Part model, mm, in its own coordinate system. Face numbers are marked on the shaded views. A direction names the side the tool comes from. Give positions to 0.01 mm unless a question says otherwise; leave off trailing zeros. Write each loop counter-clockwise with the first axis right and the second up, starting at its lowest first coordinate (ties: lowest second). Pieces come first, ordered by that corner, then holes. Notation, with made-up numbers: (-35.5, -25) - (21.5, -25) arc R25 ccw to (21.5, 11) - close; hole circle Ø3 at (-13.5, -28.5). An arc over 180 degrees is marked (long way). Answer as a JSON object with one key per item and string values. Group by question number.
```python
from build123d import *

# Parameters (mm, degrees)
SKETCH_1_R               = 20
EXTRUDE_1_DEPTH          = 5
SKETCH_1_7_R             = 3
EXTRUDE_2_DEPTH          = 10
SKETCH_2_R               = 0.75
CUT_EXTRUDE_1_DEPTH      = 31
PATTERN_CIRCULAR_1_COUNT = 6


with BuildPart() as part:
    # Sketch 1 → Extrude 1 (new body)
    with BuildSketch(Plane(origin=(0, 0, 0), x_dir=(1, 0, 0), z_dir=(0, 1, 0))):
        with Locations(Location((0, 0, 0), (0, 0, 270))):
            Circle(SKETCH_1_R)
    extrude(amount=EXTRUDE_1_DEPTH)

    # Sketch 1_7 → Extrude 2 (add)
    with BuildSketch(Plane(origin=(0, 0, 0), x_dir=(1, 0, 0), z_dir=(0, 1, 0))):
        with Locations(Location((0, 0, 0), (0, 0, 270))):
            Circle(SKETCH_1_7_R)
        with BuildLine():
            Line((-1, -1.118033989), (-1, 1.118033989))
            ThreePointArc((-1, 1.118033989), (1.5, 0), (-1, -1.118033989))
        make_face(mode=Mode.SUBTRACT)
    extrude(amount=EXTRUDE_2_DEPTH)

    # Sketch 2 → Cut-Extrude 1 (cut, through all)
    with BuildSketch(Plane.XZ):
        with Locations(Location((0, -7, 0), (0, 0, 270))):
            Circle(SKETCH_2_R)
        with Locations(Location((0, -17, 0), (0, 0, 270))):
            Circle(SKETCH_2_R)
    cut_extrude_1 = extrude(amount=-CUT_EXTRUDE_1_DEPTH, mode=Mode.SUBTRACT)

    # Pattern Circular 1: Cut-Extrude 1 ×6 about axis
    pattern_circular_1_axis = Axis((0, 0, 0), (0, 1, 0))
    for i in range(1, PATTERN_CIRCULAR_1_COUNT):
        add(cut_extrude_1.rotate(pattern_circular_1_axis, i * 360 / PATTERN_CIRCULAR_1_COUNT), mode=Mode.SUBTRACT)


solid = part.part
```
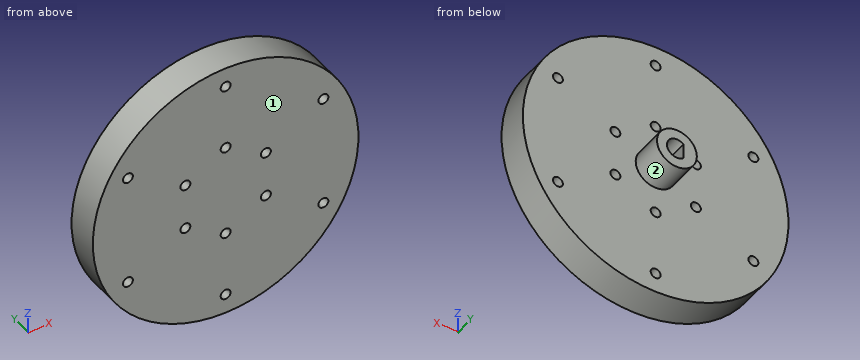
1) Saw through at D-D (z = -0.5). List the corners of the cut face in (x, y), and give its area (3 significant figures).
2) Drop flat-ended pins along their axis: P1, Ø5, axis at y = 5, z = -13.5, coming from the +X side; P2, Ø0.9, axis at x = 14.72, z = 8.5, coming from the -Y side; P3, Ø2, axis at x = -5, z = -8, coming from the +Y side; P4, Ø5, axis at x = -15, y = 5, coming from the +Z side. Give the stop position or say it passes through.
3) Saw through at B-B (y = 9.25). List the corners of the cut face in (x, z).
4) Drill centre lines: line 1 along Z through (x, y) = (0, 7.55); line 2 along X through (y, z) = (3.7, -8.5); line 3 along Y through (x, z) = (-8.5, 8.5). Where is each one in solid material? Low to high. Write a range as from..to.
5) Which spindle directions (+Z, -Z, +X, -X, +Y, -Y) get a long thin tool onto all of the face, cutting with end or side? Do the marked faces 1 and 2. Say none if no direction does.
6) Saw through at A-A (z = 7). List the corners of the cut face in (x, y) (3 decimals).
7) Saw through at C-C (y = 1.5). State how many separate pieces and enclosed holes the cut face has, and give its area (3 significant figures).
Checks:
{
 "1": {"outline": "(-19.99, 0) - (19.99, 0) - (19.99, 5) - (2.96, 5) - (2.96, 10) - (1.41, 10) - (1.41, 5) - (-1, 5) - (-1, 10) - (-2.96, 10) - (-2.96, 5) - (-19.99, 5) - close", "area": "217 mm2"},
 "2": {"P1": "x = 16.7", "P2": "through", "P3": "y = 5", "P4": "z = 15.61"},
 "3": {"outline": "circle Ø6 at (0, 0); hole (-1, -1.12) arc R1.5 ccw (long way) to (-1, 1.12) - close"},
 "4": {"line 1": "-3..-1.5, 1.5..3", "line 2": "-18.1..-15.47, -13.97..13.97, 15.47..18.1", "line 3": "0..5"},
 "5": {"face 1": "+Z, -Z, +X, -X, -Y", "face 2": "+Y"},
 "6": {"outline": "(-18.735, 0) - (-0.75, 0) - (-0.75, 5) - (-18.735, 5) - close; (0.75, 0) - (18.735, 0) - (18.735, 5) - (0.75, 5) - close"},
 "7": {"separate pieces": "1", "enclosed holes": "12", "area": "1,240 mm2"}
}
